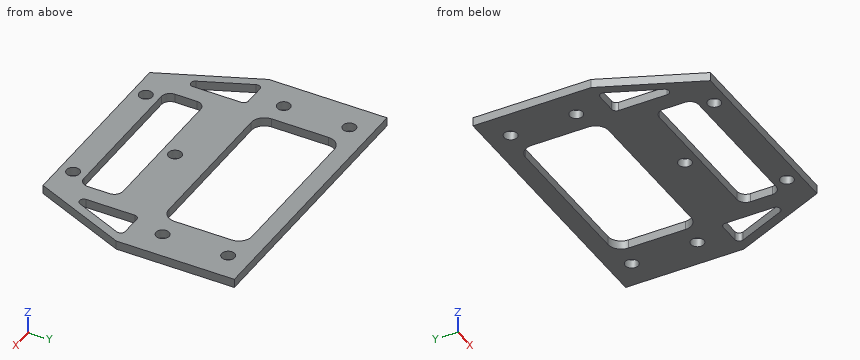
from build123d import *

# Parameters (mm, degrees)
SKETCH_1_R      = 1.5
SKETCH_1_W      = 40
SKETCH_1_H      = 19
SKETCH_1_W_2    = 36
SKETCH_1_H_2    = 9
EXTRUDE_1_DEPTH = 2
EXTRUDE_2_DEPTH = 2
FILLET_1_R      = 3
FILLET_2_R      = 2
FILLET_3_R      = 1


with BuildPart() as part:
    # 草图1 → 凸台-拉伸1 (new body)
    with BuildSketch(Plane.XY):
        Polygon((-31.5, -2), (-22, -2), (-22, -24), (22, -24), (22, -2), (31.5, -2), (31.5, 25), (-31.5, 25), align=None)
        with Locations((-25, 20)):
            Circle(SKETCH_1_R, mode=Mode.SUBTRACT)
        with Locations((25, 20)):
            Circle(SKETCH_1_R, mode=Mode.SUBTRACT)
        with Locations((-25, 5)):
            Circle(SKETCH_1_R, mode=Mode.SUBTRACT)
        with Locations((25, 5)):
            Circle(SKETCH_1_R, mode=Mode.SUBTRACT)
        with Locations((0, -6)):
            Circle(SKETCH_1_R, mode=Mode.SUBTRACT)
        with Locations((-15, -21)):
            Circle(SKETCH_1_R, mode=Mode.SUBTRACT)
        with Locations((15, -21)):
            Circle(SKETCH_1_R, mode=Mode.SUBTRACT)
        with Locations((0, 11.5)):
            Rectangle(SKETCH_1_W, SKETCH_1_H, mode=Mode.SUBTRACT)
        with Locations((0, -13.5)):
            Rectangle(SKETCH_1_W_2, SKETCH_1_H_2, mode=Mode.SUBTRACT)
    extrude(amount=EXTRUDE_1_DEPTH)

    # 草图2 → 凸台-拉伸2 (add)
    with BuildSketch(Plane.XY.offset(2)):
        Polygon((-31.5, -2), (-22, -24), (-22, -18.955049698), (-29.321498733, -2), align=None)
        Polygon((31.5, -2), (22, -24), (22, -18.955049698), (29.321498733, -2), align=None)
    extrude(amount=-EXTRUDE_2_DEPTH)

    # 圆角1
    fillet_1_edges = [part.edges().sort_by_distance(p)[0] for p in [
        (20, 2, 1),
        (20, 21, 1),
        (-20, 21, 1),
        (-20, 2, 1),
    ]]
    fillet(fillet_1_edges, radius=FILLET_1_R)

    # 圆角2
    fillet_2_edges = [part.edges().sort_by_distance(p)[0] for p in [
        (18, -18, 1),
        (18, -9, 1),
        (-18, -9, 1),
        (-18, -18, 1),
    ]]
    fillet(fillet_2_edges, radius=FILLET_2_R)

    # 圆角3
    fillet_3_edges = [part.edges().sort_by_distance(p)[0] for p in [
        (22, -2, 1),
        (-22, -2, 1),
        (-22, -18.955049698, 1),
        (-29.321498733, -2, 1),
        (22, -18.955049698, 1),
        (29.321498733, -2, 1),
    ]]
    fillet(fillet_3_edges, radius=FILLET_3_R)


solid = part.part
Model file for the job. Use its own axes, mm. Coordinates: 2 decimals unless noted, no trailing zeros. Order: outer loops, then holes, each group sorted by start corner. A loop starts at its lowest first (then second) coordinate and runs counter-clockwise, first axis right, second up. Notation, with made-up numbers: M 6,48 L 61,48 A37 cw 61,85 Z; hole C 29.25,16 d9. An arc over 180 degrees is marked long. Return JSON: item names as keys, results as strings.
1. Saw through at B-B (y = 10). Give the cut face in (x, z), and give its area (3 significant figures).
Ans:
{"outline": "M -31.5,0 L -20,0 L -20,2 L -31.5,2 Z; M 20,0 L 31.5,0 L 31.5,2 L 20,2 Z", "area": "46.0 mm^2"}
2. Saw through at C-C (y = -12.5). Give the cut face in (x, z), and give its area (3 significant figures).
Ans:
{"outline": "M -26.97,0 L -24.79,0 L -24.79,2 L -26.97,2 Z; M -22,0 L -18,0 L -18,2 L -22,2 Z; M 18,0 L 22,0 L 22,2 L 18,2 Z; M 24.79,0 L 26.97,0 L 26.97,2 L 24.79,2 Z", "area": "24.7 mm^2"}
3. Saw through at D-D (y = -21). Give the cut face in (x, z), and give its area (3 significant figures).
Ans:
{"outline": "M -23.3,0 L -16.5,0 L -16.5,2 L -23.3,2 Z; M -13.5,0 L 13.5,0 L 13.5,2 L -13.5,2 Z; M 16.5,0 L 23.3,0 L 23.3,2 L 16.5,2 Z", "area": "81.2 mm^2"}
4. Saw through at A-A (x = 9). Give the cut face in (y, z).
Ans:
{"outline": "M -24,0 L -18,0 L -18,2 L -24,2 Z; M -9,0 L 2,0 L 2,2 L -9,2 Z; M 21,0 L 25,0 L 25,2 L 21,2 Z"}
5. Drill centre lines: probe 1 along Y at (x, z) = (2, 0.2); probe 2 along Y at (x, z) = (-15, 0.9); probe 3 along X at (y, z) = (6, 1.4). Where is each one in solid material? Low to high.
Ans:
{"probe 1": "-24 to -18, -9 to 2, 21 to 25", "probe 2": "-24 to -22.5, -19.5 to -18, -9 to 2, 21 to 25", "probe 3": "-31.5 to -26.12, -23.88 to -20, 20 to 23.88, 26.12 to 31.5"}
